Could you check a few things on this model? Use its own coordinates, in mm. Face numbers are marked on the shaded views. A direction names the side the tool comes from. Round coordinates to 2 decimals unless told otherwise and drop trailing zeros. Order: outer loops, then holes, each group sorted by start corner. A loop starts at its lowest first (then second) coordinate and runs counter-clockwise, first axis right, second up. Notation, with made-up numbers: (75, 45.5) - (126, 45.5) arc R26 ccw to (126, 72.5) - close; hole circle Ø8 at (11.5, -37). An arc over 180 degrees is marked (long way). Use one line per item in the form item = value.
Solid Edge part; units mm, degrees
sketch "Sketch1" plane through (0, 0, 0) normal (0, 0, 1) x (1, 0, 0)
  line L0 (0, 46.5) -> (100, 34.83)
  line L1 (100, 34.83) -> (144.5, 5.165)
  line L2 (144.4988, -5.585) -> (144.5, 5.165)
  line L3 (126.4988, -5.585) -> (144.4988, -5.585)
  line L4 (144.5, -6.085) -> (126.4988, -6.085)
  line L5 (144.5, -6.085) -> (144.5, -16.835)
  line L6 (144.5, -16.835) -> (126.5, -34.835)
  line L7 (0, -46.5) -> (100, -46.5)
  line L8 (0, -46.5) -> (-100, -46.5)
  arc A0 (-100, -46.5) -> (-126.5, -34.835) centre (-101.022, -12.8884) cw
  line L9 (-144.5, -16.835) -> (-126.5, -34.835)
  line L10 (-144.5, -6.085) -> (-144.5, -16.835)
  line L11 (-144.5, -6.085) -> (-126.4988, -6.085)
  arc A1 (-126.4988, -6.085) -> (-126.4988, -5.585) centre (-100, -5.835) ccw
  line L12 (-126.4988, -5.585) -> (-144.4988, -5.585)
  line L13 (-144.4988, -5.585) -> (-144.5, 5.165)
  line L14 (-100, 34.83) -> (-144.5, 5.165)
  line L15 (0, 46.5) -> (-100, 34.83)
  arc A2 (126.4988, -5.585) -> (126.4988, -6.085) centre (100, -5.835) ccw
  arc A3 (126.5, -34.835) -> (100, -46.5) centre (101.022, -12.8884) cw
extrude "Protrusion1" add sketch "Sketch1" along normal blind 20
hole "Hole_1" at (139.5, 5.1649, 5) direction (0, -1, 0) diameter 6.647 end through all counterbore diameter 8.135 counterbore depth 10 thread major 8 thread length 2
hole "Hole1" at (139.5, 5.1649, 15) direction (0, -1, 0) diameter 6.647 end through all counterbore diameter 8.135 counterbore depth 10 thread major 8 thread length 2
hole "Hole2" at (-139.5, 5.158, 5) direction (0, -1, 0) diameter 6.647 end through all counterbore diameter 8.135 counterbore depth 10 thread major 8 thread length 2
hole "Hole3" at (-139.5, 5.158, 15) direction (0, -1, 0) diameter 6.647 end through all counterbore diameter 8.135 counterbore depth 10 thread major 8 thread length 2
hole "Hole_5" at (139.5, 5.1649, 15) direction (0, 1, 0) diameter 8.135 end up to next
hole "Hole4" at (139.5, 5.1649, 5) direction (0, 1, 0) diameter 8.135 end up to next
hole "Hole5" at (-139.5, 5.158, 15) direction (0, 1, 0) diameter 8.135 end up to next
hole "Hole6" at (-139.5, 5.158, 5) direction (0, 1, 0) diameter 8.135 end up to next
hole "Hole_9" at (0, 23, 0) direction (0, 0, 1) diameter 23.5 end up to next
sketch "Sketch2" plane through (0, -0.0078, 0) normal (0, 0, -1) x (1, 0, 0)
  circle A0 centre (45, -11.5078) radius 17
  circle A1 centre (-45, -11.5078) radius 17
extrude "ExtrudedProtrusion_4" add sketch "Sketch2" against normal blind 40.4
hole "Hole_10" at (-45, 11.5, 40.4) direction (0, 0, -1) diameter 10 end up to next
hole "Hole7" at (45, 11.5, 40.4) direction (0, 0, -1) diameter 10 end up to next
fillet "Round_2" radius 4.5 1 edges at (28, 11.5, 40.4)
fillet "Round_2" radius 5 1 edges at (-62, 11.5, 40.4)
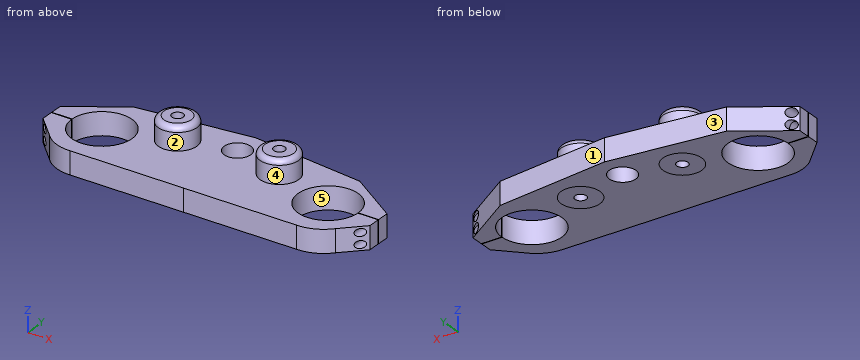
Item 1: Imagine slicing it at A-A on x = 139.5. State how many separate pieces and enclosed holes the cut face has, plus the area to 3 significant figures.
Found:
separate_pieces = 6
enclosed_holes = 0
area = 160 mm2
Item 2: Imagine slicing it at C-C on x = -45. Please give me the cut outline in (y, z).
Found:
outline = (-46.5, 0) - (6.5, 0) - (6.5, 40.4) - (-0.5, 40.4) arc R5 ccw to (-5.5, 35.4) - (-5.5, 20) - (-46.5, 20) - close; (16.5, 0) - (41.25, 0) - (41.25, 20) - (28.5, 20) - (28.5, 35.4) arc R5 ccw to (23.5, 40.4) - (16.5, 40.4) - close
Item 3: Will these pins go through, and if not, where does the flat tip stop? P1, Ø1, axis at y = 6.5, z = 25.5, coming from the +X side; P2, Ø5, axis at x = -64.5, y = -24.5, coming from the +Z side; P3, Ø10, axis at x = -24, z = 13, coming from the +Y side; P4, Ø5.5, axis at x = 139.5, z = 5, coming from the -Y side.
Found:
P1 = 61.39
P2 = 20
P3 = 44.28
P4 = through
Item 4: Imagine slicing it at B-B on z = 23.5. Please give me the cut outline in (x, y), plus the area to 3 significant figures.
Found:
outline = circle Ø34 at (-45, 11.5); circle Ø34 at (45, 11.5); hole circle Ø10 at (-45, 11.5); hole circle Ø10 at (45, 11.5)
area = 1,660 mm2
Item 5: If we mould it in two halves opening along X, with no side actions, what happens to the marked faces 1, 2 and 3? For each: released by +X, released by -X, zero draft, split by the parting line, or undercut.
Found:
face_1 = released by +X
face_2 = undercut
face_3 = released by -X
Item 6: For the marked faces 4 and 5, which set-ups out of +Z, -Z, +X, -X, +Y, -Y let a thin tool reach every point of the face, with its end or its side?
Found:
face_4 = +Z
face_5 = +Z, -Z
Item 7: I need wall thicknesses on L1, parallel to Z at x = -139.5, y = -17.5; L2, parallel to X at y = 3, z = 5; L3, parallel to Z at x = 139, y = 0. Which ranges of each line are inside material? Lowest first, please.
Found:
L1 = 0 to 1.68, 8.32 to 11.68, 18.32 to 20
L2 = -144.5 to -143.57, -135.43 to -124.98, -75.02 to 75.02, 124.98 to 135.43, 143.57 to 144.5
L3 = 0 to 0.96, 9.04 to 10.96, 19.04 to 20
